Model file for the job. Use its own axes, mm. A direction names the side the tool comes from. Give positions to 0.01 mm unless a question says otherwise; leave off trailing zeros. Write each loop counter-clockwise with the first axis right and the second up, starting at its lowest first coordinate (ties: lowest second). Pieces come first, ordered by that corner, then holes.
```python
from build123d import *

# Parameters (mm, degrees)
SKETCH1_W           = 15.2
SKETCH1_H           = 2.27
BOSS_EXTRUDE1_DEPTH = 3.8
SKETCH2_W           = 0.548157429
SKETCH2_H           = 0.54815743
SKETCH2_2_W         = 0.548157429
SKETCH2_2_H         = 0.54815743
BOSS_EXTRUDE2_DEPTH = 8.65


with BuildPart() as part:
    # Sketch1 → Boss-Extrude1 (new body)
    with BuildSketch(Plane(origin=(0, 0, 0), x_dir=(1, 0, 0), z_dir=(0, 1, 0))):
        with Locations((7.6, 1.135)):
            Rectangle(SKETCH1_W, SKETCH1_H)
    extrude(amount=BOSS_EXTRUDE1_DEPTH)

    # Sweep1: sweep along a path in Sketch3
    with BuildLine(Plane(origin=(0, 0, 0), x_dir=(0, 0, -1), z_dir=(1, 0, 0))) as sweep1_path:
        Line((2.27, 1.9), (4.07, 1.9))
        ThreePointArc((4.07, 1.9), (4.282132034, 1.812132034), (4.37, 1.6))
        Line((4.37, 1.6), (4.37, -2.4))
    # Sketch2 → Sweep1 (sweep)
    with BuildSketch(Plane(origin=(0, 0, -2.27), x_dir=(-1, 0, 0), z_dir=(0, 0, -1))):
        with Locations((-1.266407872, 1.9)):
            Rectangle(SKETCH2_W, SKETCH2_H)
        with Locations((-3.806407872, 1.9)):
            Rectangle(SKETCH2_W, SKETCH2_H)
        with Locations((-6.346407872, 1.9)):
            Rectangle(SKETCH2_W, SKETCH2_H)
        with Locations((-8.886407872, 1.9)):
            Rectangle(SKETCH2_W, SKETCH2_H)
        with Locations((-11.426407872, 1.9)):
            Rectangle(SKETCH2_W, SKETCH2_H)
        with Locations((-13.966407872, 1.9)):
            Rectangle(SKETCH2_W, SKETCH2_H)
    sweep(path=sweep1_path.line)

    # Sketch2_2 → Boss-Extrude2 (add)
    with BuildSketch(Plane(origin=(0, 0, -2.27), x_dir=(-1, 0, 0), z_dir=(0, 0, -1))):
        with Locations((-1.266407872, 1.9)):
            Rectangle(SKETCH2_2_W, SKETCH2_2_H)
        with Locations((-3.806407872, 1.9)):
            Rectangle(SKETCH2_2_W, SKETCH2_2_H)
        with Locations((-6.346407872, 1.9)):
            Rectangle(SKETCH2_2_W, SKETCH2_2_H)
        with Locations((-8.886407872, 1.9)):
            Rectangle(SKETCH2_2_W, SKETCH2_2_H)
        with Locations((-11.426407872, 1.9)):
            Rectangle(SKETCH2_2_W, SKETCH2_2_H)
        with Locations((-13.966407872, 1.9)):
            Rectangle(SKETCH2_2_W, SKETCH2_2_H)
    extrude(amount=-BOSS_EXTRUDE2_DEPTH)


solid = part.part
```
1. Pin check, flat tips, straight feed: P1, Ø1.9, axis at y = 1, z = -3, coming from the -X side; P2, Ø0.6, axis at x = 1.5, z = -3.5, coming from the -Y side; P3, Ø1.9, axis at y = 0.5, z = -4, coming from the -X side. Stop position of each tip, or through.
Calculated:
P1: stops at x = 0
P2: stops at y = 1.63
P3: stops at x = 0.99
2. Slice it at A-A, the plane y = -1.5. Write the cut outline in (x, z), and give its area (3 significant figures).
Calculated:
outline: (0.99, -4.64) - (1.54, -4.64) - (1.54, -4.1) - (0.99, -4.1) - close; (3.53, -4.64) - (4.08, -4.64) - (4.08, -4.1) - (3.53, -4.1) - close; (6.07, -4.64) - (6.62, -4.64) - (6.62, -4.1) - (6.07, -4.1) - close; (8.61, -4.64) - (9.16, -4.64) - (9.16, -4.1) - (8.61, -4.1) - close; (11.15, -4.64) - (11.7, -4.64) - (11.7, -4.1) - (11.15, -4.1) - close; (13.69, -4.64) - (14.24, -4.64) - (14.24, -4.1) - (13.69, -4.1) - close
area: 1.80 mm2
3. Slice it at C-C, the plane y = 0.5. Write the cut outline in (x, z), and give its area (3 significant figures).
Calculated:
outline: (0, -2.27) - (15.2, -2.27) - (15.2, 0) - (0, 0) - close; (0.99, -4.64) - (1.54, -4.64) - (1.54, -4.1) - (0.99, -4.1) - close; (3.53, -4.64) - (4.08, -4.64) - (4.08, -4.1) - (3.53, -4.1) - close; (6.07, -4.64) - (6.62, -4.64) - (6.62, -4.1) - (6.07, -4.1) - close; (8.61, -4.64) - (9.16, -4.64) - (9.16, -4.1) - (8.61, -4.1) - close; (11.15, -4.64) - (11.7, -4.64) - (11.7, -4.1) - (11.15, -4.1) - close; (13.69, -4.64) - (14.24, -4.64) - (14.24, -4.1) - (13.69, -4.1) - close
area: 36.3 mm2
4. Slice it at B-B, the plane z = 0.5. Write the cut outline in (x, y), and give its area (3 significant figures).
Calculated:
outline: (0.99, 1.63) - (1.54, 1.63) - (1.54, 2.17) - (0.99, 2.17) - close; (3.53, 1.63) - (4.08, 1.63) - (4.08, 2.17) - (3.53, 2.17) - close; (6.07, 1.63) - (6.62, 1.63) - (6.62, 2.17) - (6.07, 2.17) - close; (8.61, 1.63) - (9.16, 1.63) - (9.16, 2.17) - (8.61, 2.17) - close; (11.15, 1.63) - (11.7, 1.63) - (11.7, 2.17) - (11.15, 2.17) - close; (13.69, 1.63) - (14.24, 1.63) - (14.24, 2.17) - (13.69, 2.17) - close
area: 1.80 mm2
5. Probe probe 1 along Z at (x, y) = (1.25, 0.25); probe 2 along Z at (x, y) = (10.25, 1.75); probe 3 along Y at (x, z) = (9, -3.5). List the from-to ranges inside material, lowest first.
Calculated:
probe 1: z = -4.64 to -4.1, -2.27 to 0
probe 2: z = -2.27 to 0
probe 3: y = 1.63 to 2.17
6. Which spindle directions (+Z, -Z, +X, -X, +Y, -Y) get a long thin tool onto all of the face, cutting with end or side? Do faces 1 (the flat face through (11.152, 0.6, -4.3)), 2 (the flat face through (0, 2, -1)), 3 (the flat face through (14.24, 0.2, -4.3)), 4 (the flat face through (0.992, 0.6, -4.3)), 5 (the flat face through (15.2, 2, -1)). Say none if no direction does.
Calculated:
face 1: -Z, +Y, -Y
face 2: +Z, -Z, -X, +Y, -Y
face 3: -Z, +X, +Y, -Y
face 4: -Z, -X, +Y, -Y
face 5: +Z, -Z, +X, +Y, -Y
